Source: CAD feature listing. Evaluate the final solid. Frame: model axes, mm. A direction names the side the tool comes from. Round coordinates to 2 decimals unless told otherwise and drop trailing zeros. Write each loop counter-clockwise with the first axis right and the second up, starting at its lowest first coordinate (ties: lowest second). Pieces come first, ordered by that corner, then holes.
from build123d import *

# Parameters (mm, degrees)
SKETCH_1_W          = 20
SKETCH_1_H          = 14.7
SKETCH_1_R          = 1.25
EXTRUDE_1_DEPTH     = 1
SKETCH_2_W          = 7.6
SKETCH_2_H          = 5.9
EXTRUDE_2_DEPTH     = 3.2
SKETCH_3_W          = 2.93
SKETCH_3_H          = 0.9
EXTRUDE_3_DEPTH     = 3.2
CUT_EXTRUDE_START   = -0.9
CUT_EXTRUDE_1_DEPTH = 0.9
SKETCH_5_W          = 2
SKETCH_5_H          = 1.75
SKETCH_5_W_2        = 1.5
SKETCH_5_H_2        = 1.5
SKETCH_5_W_3        = 3.3
SKETCH_5_H_3        = 1.6
EXTRUDE_4_DEPTH     = 0.7
SKETCH_6_W          = 1.7
SKETCH_6_H          = 6.5
EXTRUDE_5_DEPTH     = 2.5
SKETCH_7_W          = 5.8
SKETCH_7_H          = 7.6
EXTRUDE_6_DEPTH     = 3.25
SKETCH_8_W          = 0.98
SKETCH_8_H          = 5
EXTRUDE_7_DEPTH     = 8
SKETCH_9_W          = 1.7
SKETCH_9_H          = 5.5
EXTRUDE_8_DEPTH     = 6.7


with BuildPart() as part:
    # 草图1 → 凸台-拉伸1 (new body)
    with BuildSketch(Plane(origin=(0, 0, 0), x_dir=(1, 0, 0), z_dir=(0, 1, 0))):
        with Locations((0, -2.45)):
            Rectangle(SKETCH_1_W, SKETCH_1_H)
        with Locations((-7.5, 0)):
            Circle(SKETCH_1_R, mode=Mode.SUBTRACT)
        with Locations((7.5, 0)):
            Circle(SKETCH_1_R, mode=Mode.SUBTRACT)
    extrude(amount=EXTRUDE_1_DEPTH)

    # 草图2 → 凸台-拉伸2 (add)
    with BuildSketch(Plane(origin=(0, 1, 0), x_dir=(1, 0, 0), z_dir=(0, 1, 0))):
        with Locations((-0.8, 1.45)):
            Rectangle(SKETCH_2_W, SKETCH_2_H)
    extrude(amount=EXTRUDE_2_DEPTH)

    # 草图3 → 凸台-拉伸3 (add)
    with BuildSketch(Plane(origin=(0, 0, -4.4), x_dir=(-1, 0, 0), z_dir=(0, 0, -1))):
        with Locations((0.8, 2.6)):
            Rectangle(SKETCH_3_W, SKETCH_3_H)
    extrude(amount=EXTRUDE_3_DEPTH)

    # 草图4 → 切除-拉伸1 (cut)
    with BuildSketch(Plane(origin=(0, 3.05, 0), x_dir=(1, 0, 0), z_dir=(0, 1, 0)).offset(CUT_EXTRUDE_START)):
        Polygon((-0.8, 7.6), (-2.265, 4.4), (-2.265, 7.6), (-2.265, 7.984995913), (0.665, 7.984995913), (0.665, 7.6), (0.665, 4.4), align=None)
    extrude(amount=CUT_EXTRUDE_1_DEPTH, mode=Mode.SUBTRACT)

    # 草图5 → 凸台-拉伸4 (add)
    with BuildSketch(Plane(origin=(0, 1, 0), x_dir=(1, 0, 0), z_dir=(0, 1, 0))):
        with Locations((4, 2.025)):
            Rectangle(SKETCH_5_W, SKETCH_5_H)
        with Locations((-5.6, 2.025)):
            Rectangle(SKETCH_5_W, SKETCH_5_H)
        with Locations((-3.85, -2.25)):
            Rectangle(SKETCH_5_W_2, SKETCH_5_H_2)
        with Locations((-0.8, -2.25)):
            Rectangle(SKETCH_5_W_2, SKETCH_5_H_2)
        with Locations((2.25, -2.25)):
            Rectangle(SKETCH_5_W_2, SKETCH_5_H_2)
        with Locations((1.35, -5.3)):
            Rectangle(SKETCH_5_W_3, SKETCH_5_H_3)
        with Locations((1.35, -7.5)):
            Rectangle(SKETCH_5_W_3, SKETCH_5_H_3)
    extrude(amount=EXTRUDE_4_DEPTH)

    # 草图6 → 凸台-拉伸5 (add)
    with BuildSketch(Plane(origin=(0, 1, 0), x_dir=(1, 0, 0), z_dir=(0, 1, 0))):
        with Locations((-3.15, -6.55)):
            Rectangle(SKETCH_6_W, SKETCH_6_H)
    extrude(amount=EXTRUDE_5_DEPTH)

    # 草图7 → 凸台-拉伸6 (add)
    with BuildSketch(Plane.XZ):
        with Locations((-2.6, 6)):
            Rectangle(SKETCH_7_W, SKETCH_7_H)
    extrude(amount=EXTRUDE_6_DEPTH)

    # 草图8 → 凸台-拉伸7 (add)
    with BuildSketch(Plane.XZ.offset(3.25)):
        with Locations((-5.01, 6)):
            Rectangle(SKETCH_8_W, SKETCH_8_H)
    extrude(amount=EXTRUDE_7_DEPTH)

    # 草图9 → 凸台-拉伸8 (add)
    with BuildSketch(Plane.XZ.offset(3.25)):
        with Locations((-3.15, 6.05)):
            Rectangle(SKETCH_9_W, SKETCH_9_H)
    extrude(amount=EXTRUDE_8_DEPTH)


solid = part.part
1) Contact query for flat-ended pins moving along their axis: P1, Ø5, axis at y = -8.5, z = 3.5, coming from the -X side; P2, Ø0.8, axis at x = -5.5, y = 1.5, coming from the +Z side; P3, Ø1.8, axis at x = 1.5, z = 5.5, coming from the +Y side. Output: stop coordinate, or through.
Taken from the geometry:
P1: stops at x = -5.5
P2: stops at z = -1.15
P3: stops at y = 1.7
2) Pull-direction query (X, two-part tool) for faces 1 (the face through (-4, 1.7, 2)), 2 (the face through (-8.75, 0.49, -0.05)), 3 (the face through (-10, 0.5, 2.6)); classes: released by +X, released by -X, zero draft, split by the parting line, or undercut.
Taken from the geometry:
face 1: zero draft
face 2: undercut
face 3: released by -X
3) Reachability of faces 4 (the face through (2, 1.7, 2)), 5 (the face through (1, 1.7, 7)), 6 (the face through (-4, 2, 7)) from +Z, -Z, +X, -X, +Y, -Y: full face, straight path, thin tool, end or side. Return the list, or none.
Taken from the geometry:
face 4: +Z, +X, -X, +Y
face 5: +Z, +X, +Y
face 6: +Z, -X, +Y
4) Section query D-D on z = -2. Return the cut outline in (x, y).
Taken from the geometry:
outline: (-10, 0) - (10, 0) - (10, 1) - (5, 1) - (5, 1.7) - (3, 1.7) - (3, 4.2) - (-4.6, 4.2) - (-4.6, 1.7) - (-6.6, 1.7) - (-6.6, 1) - (-10, 1) - close
5) Section query B-B on x = 7.5. Return the cut outline in (y, z).
Taken from the geometry:
outline: (0, -4.9) - (1, -4.9) - (1, -1.25) - (0, -1.25) - close; (0, 1.25) - (1, 1.25) - (1, 9.8) - (0, 9.8) - close
6) Material intervals for line 1 (X direction, y = 0.5, z = 0); line 2 (X direction, y = -5.5, z = 7.25); line 3 (Z direction, x = 7.5, y = 0.45), sorted ascending.
Taken from the geometry:
line 1: x = -10 to -8.75, -6.25 to 6.25, 8.75 to 10
line 2: x = -5.5 to -4.52, -4 to -2.3
line 3: z = -4.9 to -1.25, 1.25 to 9.8
7) Section query A-A on z = 0. Return the cut outline in (x, y), then the cut area to 3 significant figures.
Taken from the geometry:
outline: (-10, 0) - (-8.75, 0) - (-8.75, 1) - (-10, 1) - close; (-6.25, 0) - (6.25, 0) - (6.25, 1) - (3, 1) - (3, 4.2) - (-4.6, 4.2) - (-4.6, 1) - (-6.25, 1) - close; (8.75, 0) - (10, 0) - (10, 1) - (8.75, 1) - close
area: 39.3 mm2
8) Section query C-C on y = 0.25. Return the cut outline in (x, z).
Taken from the geometry:
outline: (-10, -4.9) - (10, -4.9) - (10, 9.8) - (-10, 9.8) - close; hole circle Ø2.5 at (-7.5, 0); hole circle Ø2.5 at (7.5, 0)
